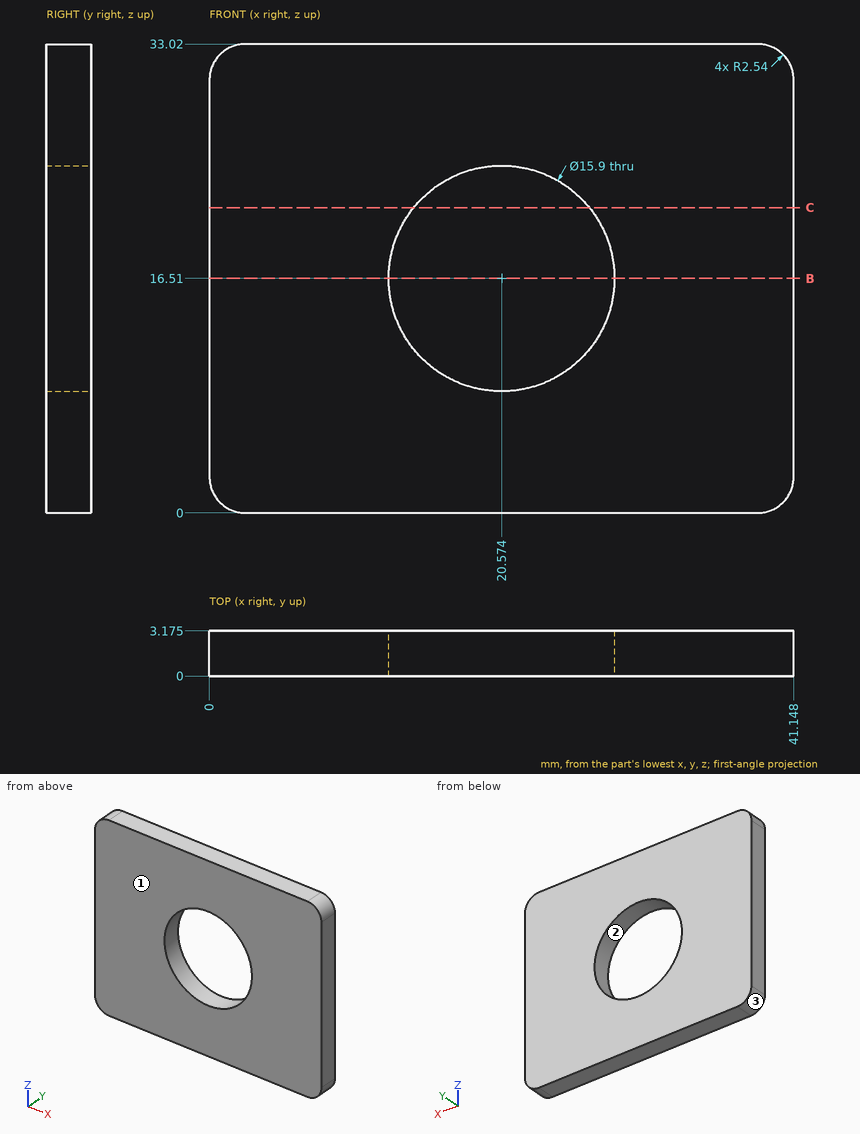
Drawing for the job (mm, zero at the part's lowest x, y, z). Round coordinates to 2 decimals unless told otherwise and drop trailing zeros. Loops run counter-clockwise (first coordinate to the right, second up) from the corner with the lowest first, then second, coordinate; pieces in that order, holes last. Notation, with made-up numbers: M -1,-4 L 43,-4 A25 cw 43,21 Z; hole C -21,8 d3. An arc over 180 degrees is marked long. Use a Markdown table: item, result. Add a question column.
(1) Pull direction Z, two halves, no side cores. Call the marked faces 1, 2 and 3: +Z half, -Z half, draft (parallel to the pull), parting line (faces both ways), or undercut.
(2) Drill centre lines: line 1 (X direction, y = 0.65, z = 16.51) (1 decimal); line 2 (Z direction, x = 22.5, y = 2.75); line 3 (Z direction, x = 23.5, y = 1.25). Where is each one in solid material? Low to high.
(3) Cut at C-C (z = 21.5). Give the cut face in (x, y) (1 decimal).
(4) Cut at B-B (z = 16.51). Give the cut face in (x, y) (1 decimal).
Geometry says:
| question | item | result |
|---|---|---|
| 1 | face 1 | draft |
| 1 | face 2 | undercut |
| 1 | face 3 | -Z half |
| 2 | line 1 | x = 0 to 12.6, 28.5 to 41.1 |
| 2 | line 2 | z = 0 to 8.8, 24.22 to 33.02 |
| 2 | line 3 | z = 0 to 9.12, 23.9 to 33.02 |
| 3 | outline | M 0,0 L 14.4,0 L 14.4,3.2 L 0,3.2 Z; M 26.8,0 L 41.1,0 L 41.1,3.2 L 26.8,3.2 Z |
| 4 | outline | M 0,0 L 12.6,0 L 12.6,3.2 L 0,3.2 Z; M 28.5,0 L 41.1,0 L 41.1,3.2 L 28.5,3.2 Z |
